Geometry check sheet. Reference: the model listing, model coordinates, mm. Coordinates: 2 decimals unless noted, no trailing zeros. Loops run counter-clockwise (first coordinate to the right, second up) from the corner with the lowest first, then second, coordinate; pieces in that order, holes last.
from build123d import *

# Parameters (mm, degrees)
SKETCH1_R           = 13.208
SKETCH1_R_2         = 3.175
BOSS_EXTRUDE4_DEPTH = 25.4
CUT_EXTRUDE3_DEPTH  = 32.528757159
CUT_EXTRUDE4_DEPTH  = 5.588


with BuildPart() as part:
    # Sketch1 → Boss-Extrude4 (new body)
    # profile 1 of 5: a face of its own
    with BuildSketch(Plane(origin=(0, 0, 0), x_dir=(1, 0, 0), z_dir=(0, 1, 0))):
        with Locations(Location((0, 0, 0), (0, 0, 270))):
            Circle(SKETCH1_R)
        Circle(SKETCH1_R_2, mode=Mode.SUBTRACT)
    # profile 2 of 5: a face of its own
    with BuildSketch(Plane(origin=(0, 0, 0), x_dir=(1, 0, 0), z_dir=(0, 1, 0))):
        with BuildLine():
            Line((1.722711816, 2.667), (0, 2.667))
            Line((0, 2.667), (-1.722711816, 2.667))
            ThreePointArc((-1.722711816, 2.667), (-1.51838977, -2.78838977), (3.175, 0))
            ThreePointArc((3.175, 0), (2.78838977, 1.51838977), (1.722711816, 2.667))
        make_face()
    # profile 3 of 5: a face of its own
    with BuildSketch(Plane(origin=(0, 0, 0), x_dir=(1, 0, 0), z_dir=(0, 1, 0))):
        with BuildLine():
            Line((-1.722711816, 2.667), (0, 2.667))
            Line((0, 2.667), (1.722711816, 2.667))
            ThreePointArc((1.722711816, 2.667), (0, 3.175), (-1.722711816, 2.667))
        make_face()
    # profile 4 of 5: a face of its own
    with BuildSketch(Plane(origin=(0, 0, 0), x_dir=(1, 0, 0), z_dir=(0, 1, 0))):
        with BuildLine():
            Line((1.722711816, 2.667), (0, 2.667))
            Line((0, 2.667), (-1.722711816, 2.667))
            ThreePointArc((-1.722711816, 2.667), (-1.51838977, -2.78838977), (3.175, 0))
            ThreePointArc((3.175, 0), (2.78838977, 1.51838977), (1.722711816, 2.667))
        make_face()
    # profile 5 of 5: a face of its own
    with BuildSketch(Plane(origin=(0, 0, 0), x_dir=(1, 0, 0), z_dir=(0, 1, 0))):
        with BuildLine():
            Line((-1.722711816, 2.667), (0, 2.667))
            Line((0, 2.667), (1.722711816, 2.667))
            ThreePointArc((1.722711816, 2.667), (0, 3.175), (-1.722711816, 2.667))
        make_face()
    extrude(amount=BOSS_EXTRUDE4_DEPTH)

    # Sketch1_6 → Cut-Extrude3 (cut, through all)
    with BuildSketch(Plane(origin=(0, 0, 0), x_dir=(1, 0, 0), z_dir=(0, 1, 0))):
        with BuildLine():
            Line((1.722711816, 2.667), (0, 2.667))
            Line((0, 2.667), (-1.722711816, 2.667))
            ThreePointArc((-1.722711816, 2.667), (-1.51838977, -2.78838977), (3.175, 0))
            ThreePointArc((3.175, 0), (2.78838977, 1.51838977), (1.722711816, 2.667))
        make_face()
    extrude(amount=CUT_EXTRUDE3_DEPTH, mode=Mode.SUBTRACT)

    # Sketch1_7 → Cut-Extrude4 (cut)
    with BuildSketch(Plane(origin=(0, 0, 0), x_dir=(1, 0, 0), z_dir=(0, 1, 0))):
        with BuildLine():
            Line((1.722711816, 2.667), (0, 2.667))
            Line((0, 2.667), (-1.722711816, 2.667))
            ThreePointArc((-1.722711816, 2.667), (-1.51838977, -2.78838977), (3.175, 0))
            ThreePointArc((3.175, 0), (2.78838977, 1.51838977), (1.722711816, 2.667))
        make_face()
        with BuildLine():
            Line((-1.722711816, 2.667), (0, 2.667))
            Line((0, 2.667), (1.722711816, 2.667))
            ThreePointArc((1.722711816, 2.667), (0, 3.175), (-1.722711816, 2.667))
        make_face()
    extrude(amount=CUT_EXTRUDE4_DEPTH, mode=Mode.SUBTRACT)


solid = part.part
(1) Draft check along Z on faces 1 (the flat face through (0, 15, -2.667)), 2 (the flat face through (3, 0, 3)), 3 (the cylindrical face through (3.967, 12.522, 12.598)). Enter one of: +Z half, -Z half, draft (parallel to the pull), parting line (faces both ways), or undercut.
Findings:
face 1: undercut
face 2: draft
face 3: parting line
(2) Sectioned sample at D-D on z = -5.75. Record the cut outline in (x, y).
Findings:
outline: (-11.89, 0) - (11.89, 0) - (11.89, 25.4) - (-11.89, 25.4) - close
(3) Sectioned sample at B-B on z = -1.75. Record the cut outline in (x, y), and give its area (3 significant figures).
Findings:
outline: (-13.09, 0) - (-2.65, 0) - (-2.65, 25.4) - (-13.09, 25.4) - close; (2.65, 0) - (13.09, 0) - (13.09, 25.4) - (2.65, 25.4) - close
area: 530 mm2
(4) Sectioned sample at A-A on x = 0. Record the cut outline in (y, z) (3 decimals), and give its area (3 significant figures).
Findings:
outline: (0, -13.208) - (25.4, -13.208) - (25.4, -2.667) - (5.588, -2.667) - (5.588, -3.175) - (0, -3.175) - close; (0, 3.175) - (25.4, 3.175) - (25.4, 13.208) - (0, 13.208) - close
area: 520 mm2
(5) Gauge pin test, flat ends, axial feed: pin 1 Ø2 at (x, y) = (9.5, 17.5) entering from +Z; pin 2 Ø3 at (y, z) = (10.5, -4.5) entering from -X; pin 3 Ø12 at (y, z) = (7.5, 9) entering from +X. Record the tip position at first contact, or that the pin passes through.
Findings:
pin 1: stops at z = 10.11
pin 2: stops at x = -12.86
pin 3: stops at x = 12.86
(6) Sectioned sample at C-C on y = 2.25. Record the cut outline in (x, z) (3 decimals), and give its area (3 significant figures).
Findings:
outline: circle Ø26.416 at (0, 0); hole circle Ø6.35 at (0, 0)
area: 516 mm2
(7) Scan lines: L1, parallel to X at y = 11.75, z = -2.25; L2, parallel to Z at x = 2, y = 16.25; L3, parallel to Z at x = 1, y = 15. Record each from-to range of solid material in increasing order.
Findings:
L1: x = -13.01 to -2.24, 2.24 to 13.01
L2: z = -13.06 to -2.47, 2.47 to 13.06
L3: z = -13.17 to -2.67, 3.01 to 13.17
